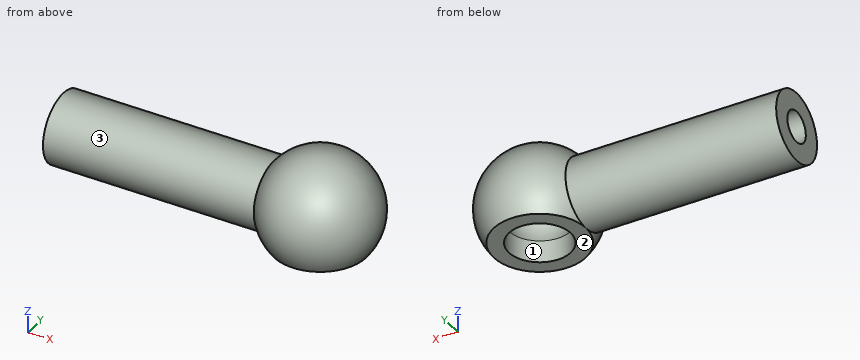
```python
from build123d import *

# Parameters (mm, degrees)
SCHIZZO2_R                    = 2.05
ESTRUSIONE_ESTRUSIONE1_DEPTH  = 13
SCHIZZO3_R                    = 0.925
TAGLIO_ESTRUSIONE1_DEPTH      = 12
TAGLIO_ESTRUSIONE2_REACH      = 21.682
TAGLIO_ESTRUSIONE2_END_RADIUS = 1.975
SCHIZZO5_R                    = 1.825


with BuildPart() as part:
    # Schizzo2 → Estrusione-Estrusione1 (new body)
    with BuildSketch(Plane(origin=(0, 0, 0), x_dir=(0, 0, -1), z_dir=(1, 0, 0))):
        with Locations(Location((0, 0, 0), (0, 0, 180))):
            Circle(SCHIZZO2_R)
    extrude(amount=ESTRUSIONE_ESTRUSIONE1_DEPTH)

    # Schizzo3 → Taglio-Estrusione1 (cut)
    with BuildSketch(Plane.ZY):
        Circle(SCHIZZO3_R)
    extrude(amount=-TAGLIO_ESTRUSIONE1_DEPTH, mode=Mode.SUBTRACT)

    # Schizzo4 → Rivoluzione1 (revolve)
    with BuildSketch(Plane(origin=(0, 0, 0), x_dir=(1, 0, 0), z_dir=(0, 1, 0))):
        with BuildLine():
            Line((15.19, 3.41), (15.19, 1.975))
            ThreePointArc((15.19, 1.975), (17.165, 0), (15.19, -1.975))
            Line((15.19, -1.975), (15.19, -3.41))
            ThreePointArc((15.19, -3.41), (18.6, 0), (15.19, 3.41))
        make_face()
    revolve(axis=Axis((15.19, 0, 1.975), (0, 0, 1)))

    # TaglioSuperficie1
    split(bisect_by=Plane(origin=(0, 0, -2.05), x_dir=(-1, 0, 0), z_dir=(0, 0, -1)), keep=Keep.BOTTOM)

    # Taglio-Estrusione2: up to this sphere (the profile starts outside it)
    taglio_estrusione2_end = Location((15.19, 0, 0)) * Sphere(TAGLIO_ESTRUSIONE2_END_RADIUS, mode=Mode.PRIVATE)
    # Schizzo5 → Taglio-Estrusione2 (cut, up to the surface)
    with BuildSketch(Plane(origin=(0, 0, -2.05), x_dir=(-1, 0, 0), z_dir=(0, 0, -1)), mode=Mode.PRIVATE) as taglio_estrusione2_sk1:
        with Locations((-15.19, 0)):
            Circle(SCHIZZO5_R)
    taglio_estrusione2_tool1 = extrude(taglio_estrusione2_sk1.sketch, amount=-TAGLIO_ESTRUSIONE2_REACH, mode=Mode.PRIVATE) - taglio_estrusione2_end
    add(taglio_estrusione2_tool1.solids().sort_by_distance((15.19, 0, -2.05))[0], mode=Mode.SUBTRACT)


solid = part.part
```
Input: part model. Units: mm. Frame: model coordinates. Face numbers are marked on the shaded views. Round coordinates to 2 decimals unless told otherwise and drop trailing zeros. Loops run counter-clockwise (first coordinate to the right, second up) from the corner with the lowest first, then second, coordinate; pieces in that order, holes last.
1) Section query A-A on z = 0. Return the cut outline in (x, y) (3 decimals), plus the area to 3 significant figures.
Ans:
outline: (0, -2.05) - (12.465, -2.05) arc R3.41 ccw (long way) to (12.465, 2.05) - (0, 2.05) - (0, 0.925) - (11.908, 0.925) arc R3.41 ccw to (11.908, -0.925) - (0, -0.925) - close; hole circle Ø3.95 at (15.19, 0)
area: 51.6 mm2
2) Section query B-B on x = 15.19. Return the cut outline in (y, z) (3 decimals).
Ans:
outline: (-2.725, -2.05) - (-1.825, -2.05) - (-1.825, -0.755) arc R1.975 cw (long way) to (1.825, -0.755) - (1.825, -2.05) - (2.725, -2.05) arc R3.41 ccw (long way) to start
3) Section query D-D on x = 5.25. Return the cut outline in (y, z) (3 decimals), plus the area to 3 significant figures.
Ans:
outline: circle Ø4.1 at (0, 0); hole circle Ø1.85 at (0, 0)
area: 10.5 mm2
4) Section query C-C on y = -1.5. Return the cut outline in (x, z) (3 decimals).
Ans:
outline: (0, -1.397) - (12.465, -1.397) arc R3.062 ccw to (12.915, -2.05) - (14.15, -2.05) - (14.15, -0.755) arc R1.285 cw (long way) to (16.23, -0.755) - (16.23, -2.05) - (17.465, -2.05) arc R3.062 ccw (long way) to (12.465, 1.397) - (0, 1.397) - close
5) Pull-direction query (Y, two-part tool) for the marked faces 1, 2 and 3; classes: released by +Y, released by -Y, zero draft, split by the parting line, or undercut.
Ans:
face 1: undercut
face 2: zero draft
face 3: split by the parting line
6) Pin query (flat end, axial travel): pin 1 (2 mm diameter, centred on x = 12.5, y = 1.5, fed in from +Z); pin 2 (2 mm diameter, centred on x = 10, z = -1, fed in from -Y); pin 3 (2 mm diameter, centred on x = 10.5, z = 1, fed in from +Y). Return the tip coordinate at first contact, or that it passes through.
Ans:
pin 1: stops at z = 2.7
pin 2: stops at y = -2.05
pin 3: stops at y = 2.05
7) Material intervals for line 1 (Y direction, x = 6.75, z = 0) (3 decimals); line 2 (Z direction, x = 5.5, y = 0.5); line 3 (X direction, y = 0, z = -1.6) (3 decimals), sorted ascending.
Ans:
line 1: y = -2.05 to -0.925, 0.925 to 2.05
line 2: z = -1.99 to -0.78, 0.78 to 1.99
line 3: x = 0 to 13.365, 17.015 to 18.201
